from build123d import *

# Parameters (mm, degrees)
F0_W     = 40.854881
F0_H     = 39.956439
F1_DEPTH = 53.121515
F2_R     = 5
F3_R     = 12.424577
F4_DEPTH = 39.957439


with BuildPart() as f1:
    # F0 (on Front) → F1 (new body)
    with BuildSketch(Plane.XZ):
        with Locations((24.789358, 34.14881)):
            Rectangle(F0_W, F0_H)
    extrude(amount=F1_DEPTH)

    # F2
    f2_edges = [f1.edges().sort_by_distance(p)[0] for p in [
        (45.216799, -26.560757, 54.12703),
        (4.361918, -26.560757, 54.12703),
        (24.789358, 0, 54.12703),
        (24.789358, -53.121515, 54.12703),
    ]]
    fillet(f2_edges, radius=F2_R)

    # F3 (on face) → F4 (cut, through all)
    with BuildSketch(Plane.XY.offset(54.12703)):
        with Locations((25.2368, -21.631569)):
            Circle(F3_R)
    extrude(amount=-F4_DEPTH, mode=Mode.SUBTRACT)


solid = f1.part
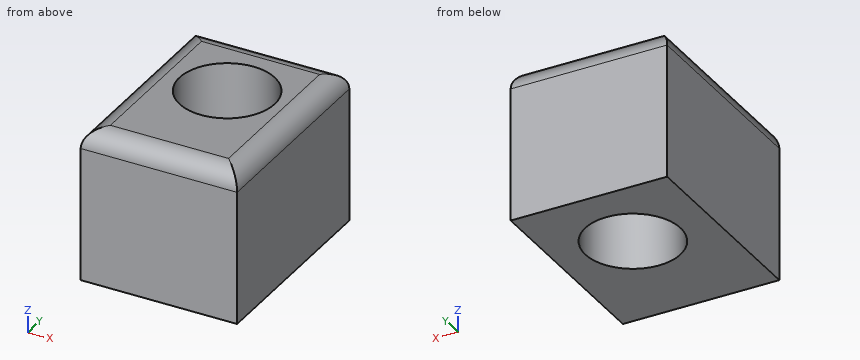
Can you work these out from the model? Positions are in its coordinate system, mm. Give positions to 0.01 mm unless a question says otherwise; leave off trailing zeros. Loops run counter-clockwise (first coordinate to the right, second up) from the corner with the lowest first, then second, coordinate; pieces in that order, holes last. Notation, with made-up numbers: (71, 87) - (87, 87) arc R3 ccw to (87, 92) - close; hole circle Ø11 at (-7, 77). An arc over 180 degrees is marked (long way). Answer as a JSON object with one key per item and string values.
Q1. Imagine slicing it at B-B on y = -13. Write out the boundary of the cut face in (x, z), plus the area to 3 significant figures.
Geometry says:
{"outline": "(4.36, 14.17) - (16.3, 14.17) - (16.3, 54.13) - (9.36, 54.13) arc R5 ccw to (4.36, 49.13) - close; (34.17, 14.17) - (45.22, 14.17) - (45.22, 49.13) arc R5 ccw to (40.22, 54.13) - (34.17, 54.13) - close", "area": "908 mm²"}
Q2. Imagine slicing it at C-C on z = 18. Write out the boundary of the cut face in (x, y).
Geometry says:
{"outline": "(4.36, -53.12) - (45.22, -53.12) - (45.22, 0) - (4.36, 0) - close; hole circle Ø24.85 at (25.24, -21.63)"}
Q3. Imagine slicing it at D-D on z = 50.5. Write out the boundary of the cut face in (x, y).
Geometry says:
{"outline": "(4.55, -52.93) - (45.02, -52.93) - (45.02, -0.19) - (4.55, -0.19) - close; hole circle Ø24.85 at (25.24, -21.63)"}
Q4. If I drill on L1, parallel to X at y = -31, z = 35.5; L2, parallel to Y at x = 30, z = 27; L3, parallel to Y at x = 28, z = 43, over which ranges is the centre line in solid material (lowest first)?
Geometry says:
{"L1": "4.36 to 17.08, 33.4 to 45.22", "L2": "-53.12 to -33.11, -10.16 to 0", "L3": "-53.12 to -33.74, -9.52 to 0"}
Q5. Imagine slicing it at A-A on x = 21. Write out the boundary of the cut face in (y, z).
Geometry says:
{"outline": "(-53.12, 14.17) - (-33.31, 14.17) - (-33.31, 54.13) - (-48.12, 54.13) arc R5 ccw to (-53.12, 49.13) - close; (-9.95, 14.17) - (0, 14.17) - (0, 49.13) arc R5 ccw to (-5, 54.13) - (-9.95, 54.13) - close"}
Q6. Will these pins go through, and if not, where does the flat tip stop? P1, Ø6, axis at x = 29, y = -15.5, coming from the +Z side (1 decimal); P2, Ø12, axis at x = 34.5, z = 38.5, coming from the +Y side.
Geometry says:
{"P1": "through", "P2": "y = 0"}
